Input: dimensioned drawing with shaded views. Units: mm. Origin: part minimum x, y, z. Round coordinates to 2 decimals unless told otherwise and drop trailing zeros. Loops run counter-clockwise (first coordinate to the right, second up) from the corner with the lowest first, then second, coordinate; pieces in that order, holes last. Notation, with made-up numbers: (-32, 15) - (22, 15) arc R34 cw to (22, 52) - close; hole circle Ø11 at (-4.75, 73). An arc over 180 degrees is marked (long way). Answer as CSV lines item,"result".
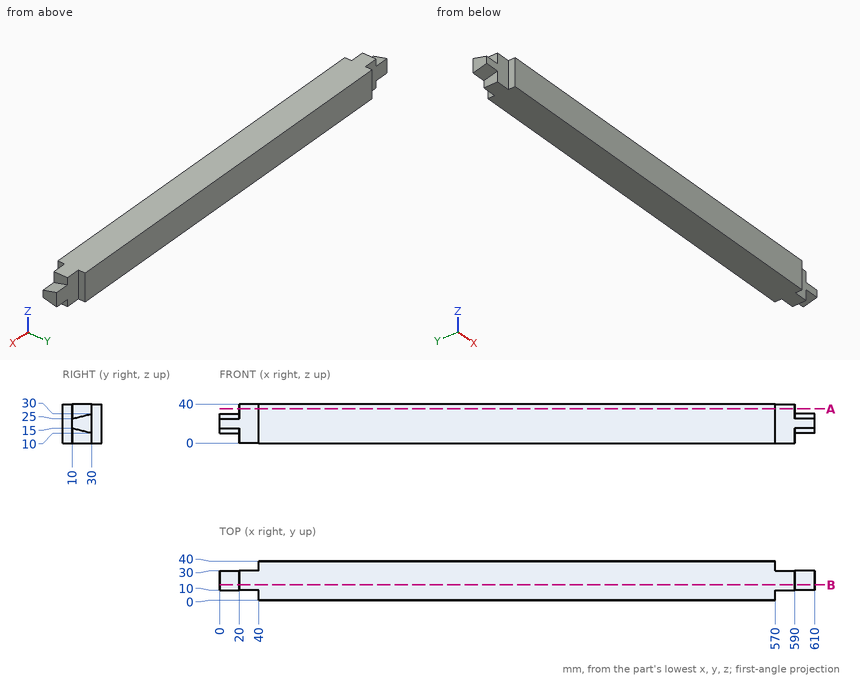
(1) Section B-B (y = 15.5). Output: boundary loops of the cut face in (x, z) (3 decimals).
Findings below:
outline,"(0, 13.625) - (20, 13.625) - (20, 0) - (590, 0) - (590, 13.625) - (610, 13.625) - (610, 26.375) - (590, 26.375) - (590, 40) - (20, 40) - (20, 26.375) - (0, 26.375) - close"
(2) Section A-A (z = 35). Output: boundary loops of the cut face in (x, y).
Findings below:
outline,"(20, 10) - (40, 10) - (40, 0) - (570, 0) - (570, 10) - (590, 10) - (590, 30) - (570, 30) - (570, 40) - (40, 40) - (40, 30) - (20, 30) - close"
(3) Pin query (flat end, axial travel): P1, Ø8, axis at y = 35.5, z = 26, coming from the +X side; P2, Ø5, axis at y = 34, z = 11.5, coming from the -X side; P3, Ø3, axis at y = 12, z = 4.5, coming from the -X side. Return the tip coordinate at first contact, or that it passes through.
Findings below:
P1,"x = 570"
P2,"x = 40"
P3,"x = 20"
(4) Material intervals for line 1 along X through (y, z) = (4.5, 26.5); line 2 along Y through (x, z) = (37.5, 29); line 3 along X through (y, z) = (20, 35), sorted ascending.
Findings below:
line 1,"40 to 570"
line 2,"10 to 30"
line 3,"20 to 590"
